```python
from build123d import *

# Parameters (mm, degrees)
CUT_EXTRUDE1_DEPTH      = 118.447860772
CUT_EXTRUDE1_DEPTH_BACK = 118.447860772
SKETCH4_W               = 55
SKETCH4_H               = 7


with BuildPart() as part:
    # Sketch1 → Revolve3 (revolve)
    with BuildSketch(Plane(origin=(0, 0, 0), x_dir=(1, 0, 0), z_dir=(0, 1, 0)), mode=Mode.PRIVATE) as revolve3_sk:
        Polygon((0, 0), (112, 0), (112, 13.5), (27, 13.5), (27, 25), (15, 25), (15, 11), (0, 11), align=None)
    revolve(revolve3_sk.sketch.rotate(Axis((0, 0, 0), (1, 0, 0)), 180), axis=Axis((0, 0, 0), (1, 0, 0)))

    # Sketch4 → Cut-Extrude1 (cut, two sides: drawn at the far end of the back side and taken through both)
    with BuildSketch(Plane(origin=(0, 0, 0), x_dir=(1, 0, 0), z_dir=(0, 1, 0)).offset(-CUT_EXTRUDE1_DEPTH_BACK)):
        with Locations((69.5, 0)):
            Rectangle(SKETCH4_W, SKETCH4_H)
    extrude(amount=CUT_EXTRUDE1_DEPTH + CUT_EXTRUDE1_DEPTH_BACK, mode=Mode.SUBTRACT)


solid = part.part
```
Model file for the job. Use its own axes, mm. A direction names the side the tool comes from. Round coordinates to 2 decimals unless told otherwise and drop trailing zeros. Write each loop counter-clockwise with the first axis right and the second up, starting at its lowest first coordinate (ties: lowest second). Pieces come first, ordered by that corner, then holes. Notation, with made-up numbers: (-31, 19) - (-12, 19) arc R34 ccw to (-12, 50) - close; hole circle Ø6 at (51.25, 64.25). An arc over 180 degrees is marked (long way). One line per item, written item: value.
(1) 3-axis set-ups, long thin cutter, end or side, ignore diameter. For faces 1 (the flat face through (0, 0, 0)), 2 (the flat face through (69, 0, -3.5)), 3 (the cylindrical face through (68.9, 5.17, 12.47)), 4 (the cylindrical face through (7.4, 10.74, -2.38)): which of +Z, -Z, +X, -X, +Y, -Y reach the whole face in a straight line?
Values follow:
face 1: +Z, -Z, -X, +Y, -Y
face 2: +Y, -Y
face 3: +X
face 4: -X
(2) Cut at A-A, the plane z = 0. Give the cut face in (x, y).
Values follow:
outline: (0, -11) - (15, -11) - (15, -25) - (27, -25) - (27, -13.5) - (42, -13.5) - (42, 13.5) - (27, 13.5) - (27, 25) - (15, 25) - (15, 11) - (0, 11) - close; (97, -13.5) - (112, -13.5) - (112, 13.5) - (97, 13.5) - close
(3) Cut at B-B, the plane y = 0. Give the cut face in (x, z), plus the area to 3 significant figures.
Values follow:
outline: (0, -11) - (15, -11) - (15, -25) - (27, -25) - (27, -13.5) - (112, -13.5) - (112, 13.5) - (27, 13.5) - (27, 25) - (15, 25) - (15, 11) - (0, 11) - close; hole (42, -3.5) - (97, -3.5) - (97, 3.5) - (42, 3.5) - close
area: 2,840 mm²
(4) Wall check: probe 1 along X at (y, z) = (6, 1); probe 2 along X at (y, z) = (-10, 6); probe 3 along X at (y, z) = (1, -16). Give the ranges that are in metal, low to high.
Values follow:
probe 1: x = 0 to 42, 97 to 112
probe 2: x = 15 to 112
probe 3: x = 15 to 27
(5) Cut at C-C, the plane x = 52.5. Give the cut face in (y, z).
Values follow:
outline: (-13.04, -3.5) arc R13.5 ccw to (13.04, -3.5) - close; (-13.04, 3.5) - (13.04, 3.5) arc R13.5 ccw to start
(6) Cut at D-D, the plane x = 10. Give the cut face in (y, z), plus the area to 3 significant figures.
Values follow:
outline: circle Ø22 at (0, 0)
area: 380 mm²
(7) Drop flat-ended pins along their axis: P1, Ø8, axis at x = 54, z = 16, coming from the -Y side; P2, Ø5, axis at y = -4.5, z = -15.5, coming from the +X side; P3, Ø10, axis at x = 58, z = -12, coming from the -Y side; P4, Ø8, axis at x = 43.5, z = -19.5, coming from the -Y side. Give the stop position or say it passes through.
Values follow:
P1: stops at y = -6.18
P2: stops at x = 27
P3: stops at y = -11.54
P4: passes through
(8) Two-plate mould, pull along X, no slides. Class faces 5 (the flat face through (27, 11, -11)), 6 (the flat face through (42, 0, 0)), 7 (the cylindrical face through (20.916, -7.509, 23.846)): pulls with the +X half, pulls with the -X half, needs draft (parallel to the pull), parting line crosses it, or undercut.
Values follow:
face 5: pulls with the +X half
face 6: undercut
face 7: needs draft
